Could you check a few things on this drawing? It's one solid part, dimensions in mm from its lowest x, y, z. A direction names the side the tool comes from. Coordinates: 2 decimals unless noted, no trailing zeros. Order: outer loops, then holes, each group sorted by start corner. A loop starts at its lowest first (then second) coordinate and runs counter-clockwise, first axis right, second up. Notation, with made-up numbers: (74, -33) -> (117, -33) arc R20 cw to (117, -6) -> close; hole circle Ø3 at (14.5, 61.5). An arc over 180 degrees is marked (long way). Answer as CSV lines item,"result".
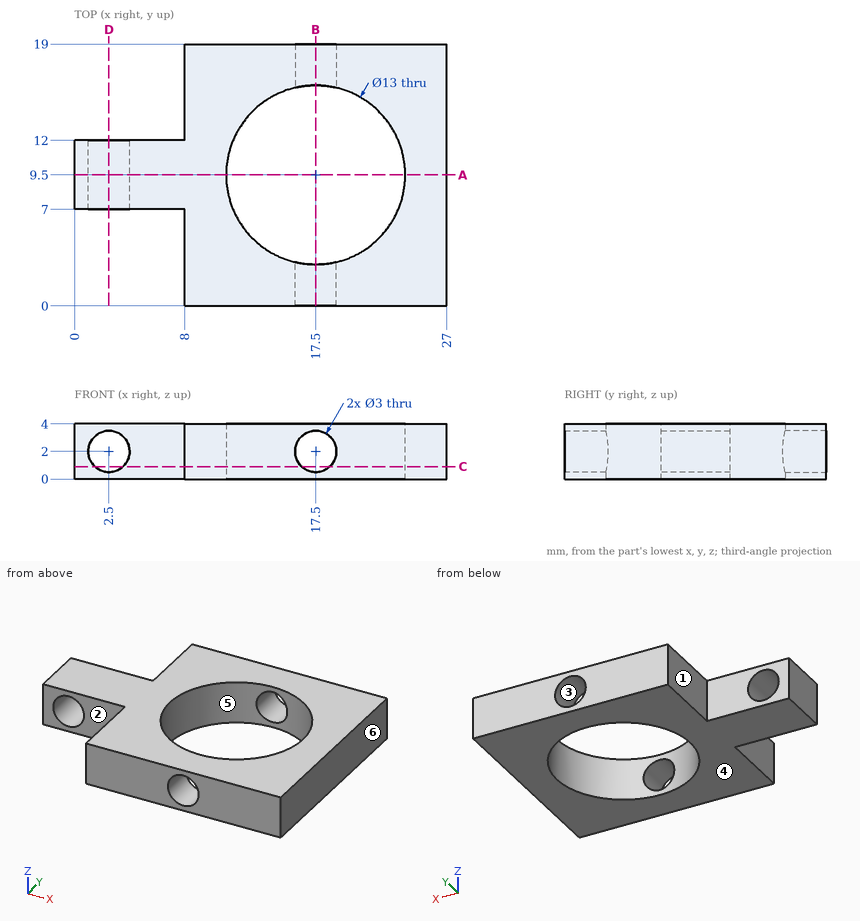
Q1. Which directions (+Z, -Z, +X, -X, +Y, -Y) give clear straight access to the entire face, cutting with the end or side of a thin tool? Please do the marked faces 1, 2 and 3.
Solution:
face 1,"+Z, -Z, -X, +Y"
face 2,"+Z, -Z, -X, -Y"
face 3,"+Y, -Y"
Q2. Imagine slicing it at B-B (x = 17.5). List the corners of the cut face in (y, z) for me.
Solution:
outline,"(0, 0) -> (3, 0) -> (3, 0.5) -> (0, 0.5) -> close; (0, 3.5) -> (3, 3.5) -> (3, 4) -> (0, 4) -> close; (16, 0) -> (19, 0) -> (19, 0.5) -> (16, 0.5) -> close; (16, 3.5) -> (19, 3.5) -> (19, 4) -> (16, 4) -> close"
Q3. For P1, Ø1.2, axis at y = 16.5, z = 1.5, coming from the -X side, with a flat end and sliding along its axis, tell me the tip position at first contact or that it passes through.
Solution:
P1,"x = 8"
Q4. We'd pull the mould along X, two halves only. Please class the marked faces 4, 5 and 6: pulls with the +X half, pulls with the -X half, needs draft (parallel to the pull), parting line crosses it, or undercut.
Solution:
face 4,"needs draft"
face 5,"undercut"
face 6,"pulls with the +X half"
Q5. Imagine slicing it at D-D (x = 2.5). List the corners of the cut face in (y, z) for me, and give its area (3 significant figures).
Solution:
outline,"(7, 0) -> (12, 0) -> (12, 0.5) -> (7, 0.5) -> close; (7, 3.5) -> (12, 3.5) -> (12, 4) -> (7, 4) -> close"
area,"5.00 mm2"
Q6. Imagine slicing it at C-C (z = 0.9). List the corners of the cut face in (x, y) for me, and give its area (3 significant figures).
Solution:
outline,"(0, 7) -> (1.48, 7) -> (1.48, 12) -> (0, 12) -> close; (3.52, 7) -> (8, 7) -> (8, 0) -> (16.48, 0) -> (16.48, 3.08) arc R6.5 cw to (16.48, 15.92) -> (16.48, 19) -> (8, 19) -> (8, 12) -> (3.52, 12) -> close; (18.52, 0) -> (27, 0) -> (27, 19) -> (18.52, 19) -> (18.52, 15.92) arc R6.5 cw to (18.52, 3.08) -> close"
area,"246 mm2"
Q7. If I drill on line 1 (Z direction, x = 2.5, y = 9.55); line 2 (X direction, y = 16.6, z = 2); line 3 (Y direction, x = 23.5, z = 1.6), over which ranges is the centre line in solid material (lowest first)?
Solution:
line 1,"0 to 0.5, 3.5 to 4"
line 2,"8 to 16, 19 to 27"
line 3,"0 to 7, 12 to 19"
Q8. Imagine slicing it at A-A (y = 9.5). List the corners of the cut face in (x, z) for me.
Solution:
outline,"(0, 0) -> (11, 0) -> (11, 4) -> (0, 4) -> close; (24, 0) -> (27, 0) -> (27, 4) -> (24, 4) -> close; hole circle Ø3 at (2.5, 2)"
